Autodesk Inventor part; units mm, degrees
ref_plane "YZ Plane" through (0, 0, 0) normal (1, 0, 0) x (0, 1, 0)
ref_plane "XZ Plane" through (0, 0, 0) normal (0, 1, 0) x (-1, 0, 0)
ref_plane "XY Plane" through (0, 0, 0) normal (0, 0, 1) x (1, 0, 0)
sketch "스케치1" plane through (0, 0, 0) normal (0, 0, 1) x (1, 0, 0)
  line L0 (-6, 5) -> (6, 5)
  line L1 (6, 5) -> (6, -5)
  line L2 (6, -5) -> (-6, -5)
  line L3 (-6, -5) -> (-6, 5)
  line L4 (-6, 5) -> (6, -5) construction
  line L5 (6, 5) -> (-6, -5) construction
  point P0 (0, 0)
  dimension "d0" = 12
  dimension "d1" = 10
extrude "돌출1" add sketch "스케치1" along normal blind 9
sketch "스케치2" plane through (0, 0, 9) normal (0, 0, 1) x (1, 0, 0)
  line L0 (-6, 5) -> (-6, -5)
  line L1 (-6, -5) -> (6, -5)
  line L2 (6, -5) -> (6, 5)
  line L3 (6, 5) -> (-6, 5)
  line L4 (-2.8796, -5) -> (2.8796, -5)
  line L5 (2.8796, -5) -> (2.8796, 5) construction
  line L6 (2.8796, 5) -> (-2.8796, 5)
  line L7 (-2.8796, 5) -> (-2.8796, -5) construction
  line L8 (-2.8796, -5) -> (2.8796, 5) construction
  line L9 (2.8796, -5) -> (-2.8796, 5) construction
  line L10 (-6, 0) -> (6, 0) construction
  arc A0 (-2.8796, 5) -> (-2.8796, -5) centre (-0.4339, 0) ccw
  arc A1 (2.8796, -5) -> (2.8796, 5) centre (0.4339, 0) ccw
  point P0 (0, 0)
extrude "돌출2" add sketch "스케치2" along normal blind 15.4 contours A0 L3 A1 L1
sketch "스케치3" plane through (0, 0, 0) normal (0, 0, -1) x (-1, 0, 0)
  circle A0 centre (0, 0) radius 2
  dimension "d6" = 4
extrude "돌출3" add sketch "스케치3" along normal blind 0.8
sketch "스케치4" plane through (0, 0, 0) normal (0, 0, -1) x (-1, 0, 0)
  circle A0 centre (0, 0) radius 1.5
  dimension "d9" = 3
extrude "돌출4" add sketch "스케치4" along normal blind 10
sketch "스케치5" plane through (0, 0, -10) normal (0, 0, -1) x (-1, 0, 0)
  circle A0 centre (0, 0) radius 1.5
  line L0 (-1.118, 1) -> (1.118, 1)
  dimension "d12" = 1
extrude "돌출5" cut sketch "스케치5" against normal blind 10 contours L0 A0 picked at (-0.0599, 1.1631)
properties part number "모터"
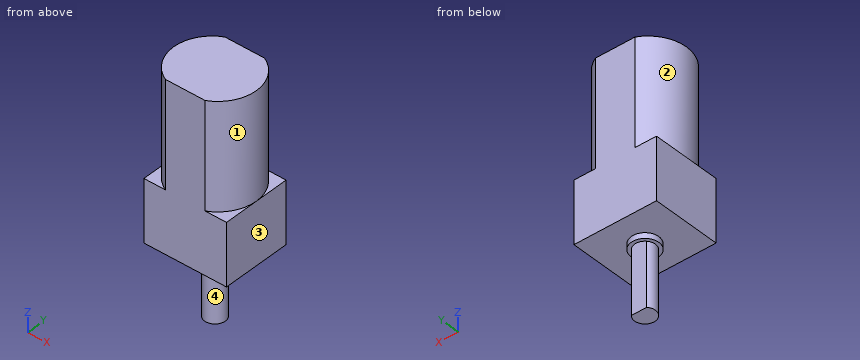
CAD build for the part. Positions are in the model's coordinates, mm. Face numbers are marked on the shaded views. A direction names the side the tool comes from. Give positions to 0.01 mm unless a question says otherwise; leave off trailing zeros. Write each loop counter-clockwise with the first axis right and the second up, starting at its lowest first coordinate (ties: lowest second). Pieces come first, ordered by that corner, then holes. Notation, with made-up numbers: (60.5, -19) - (101.5, -19) arc R29 ccw to (101.5, 2) - close; hole circle Ø2 at (27.25, 84). An arc over 180 degrees is marked (long way). Answer as CSV lines item,"result".
Q1. 3-axis set-ups, long thin cutter, end or side, ignore diameter. For the marked faces 1, 2, 3 and 4: which of +Z, -Z, +X, -X, +Y, -Y reach the whole face in a straight line?
Result set:
face 1,"+Z, +X"
face 2,"+Z, -X"
face 3,"+Z, -Z, +X, +Y, -Y"
face 4,"-Z"
Q2. Flat gauge pins, fed straight in: pin 1 Ø5 at (y, z) = (0.5, -3.5) entering from +X; pin 2 Ø1.5 at (y, z) = (3.5, 20) entering from +X; pin 3 Ø2 at (x, z) = (0.5, -6) entering from +Y. Where does each tip first touch, or does it go through?
Result set:
pin 1,"x = 1.5"
pin 2,"x = 5.27"
pin 3,"y = 1"
Q3. Drill centre lines: line 1 (Z direction, x = -5, y = 3.25); line 2 (Z direction, x = -4, y = -4); line 3 (X direction, y = -1, z = -1). Where is each one in solid material? Low to high. Write a range as from..to.
Result set:
line 1,"0..9"
line 2,"0..24.4"
line 3,"-1.12..1.12"
Q4. Band-saw the part on A-A (x = 0). Give the cut face in (y, z), and give its area (3 significant figures).
Result set:
outline,"(-5, 0) - (-2, 0) - (-2, -0.8) - (-1.5, -0.8) - (-1.5, -10) - (1, -10) - (1, 0) - (1.5, 0) - (1.5, -0.8) - (2, -0.8) - (2, 0) - (5, 0) - (5, 24.4) - (-5, 24.4) - close"
area,"270 mm²"
Q5. Band-saw the part on C-C (z = -1.5). Give the cut face in (x, y).
Result set:
outline,"(-1.12, 1) arc R1.5 ccw (long way) to (1.12, 1) - close"
Q6. Band-saw the part on D-D (x = 4.75). Give the cut face in (y, z), and give its area (3 significant figures).
Result set:
outline,"(-5, 0) - (5, 0) - (5, 9) - (3.51, 9) - (3.51, 24.4) - (-3.51, 24.4) - (-3.51, 9) - (-5, 9) - close"
area,"198 mm²"
Q7. Band-saw the part on B-B (y = 4). Give the cut face in (x, z).
Result set:
outline,"(-6, 0) - (6, 0) - (6, 9) - (4.3, 9) - (4.3, 24.4) - (-4.3, 24.4) - (-4.3, 9) - (-6, 9) - close"
